CAD build for the part. Positions are in the model's coordinates, mm. A direction names the side the tool comes from. Coordinates: 2 decimals unless noted, no trailing zeros. Write each loop counter-clockwise with the first axis right and the second up, starting at its lowest first coordinate (ties: lowest second). Pieces come first, ordered by that corner, then holes. Notation, with made-up numbers: (-14, 72.25) - (35, 72.25) arc R21 ccw to (35, 78.25) - close; hole circle Ø6 at (65.5, -5). An arc over 180 degrees is marked (long way). Answer in a Markdown table with one row per item. Add a question column.
Q1. Band-saw the part on C-C (x = 26). List the corners of the cut face in (y, z).
Q2. Band-saw the part on D-D (z = -22). List the corners of the cut face in (x, y).
Q3. 3-axis set-ups, long thin cutter, end or side, ignore diameter. For faces 1 (the flat face through (-1, -20, 1)), 2 (the flat face through (-1, 0, -39.5)): which of +Z, -Z, +X, -X, +Y, -Y reach the whole face in a straight line?
Q4. Two-plate mould, pull along Z, no slides. Class faces 3 (the flat face through (1, 3, -5)), 4 (the flat face through (1, 0, 75)), 5 (the cylindrical face through (-0.651, -10.14, -40.043)), 6 (the flat face through (75, -5, 16)): +Z half, -Z half, draft (parallel to the pull), parting line (faces both ways), or undercut.
Q5. Drill centre lines: line 1 along Z through (x, y) = (0, -4); line 2 along Z through (x, y) = (-27, 5); line 3 along Y through (x, z) = (-63, -50). Where is each one in solid material? Low to high. Write a range as from..to.
Q6. Band-saw the part on B-B (z = -45). List the corners of the cut face in (x, y), and give its area (3 significant figures).
Q7. Pin check, flat tips, straight feed: pin 1 (3 mm diameter, centred on x = 9, z = 7, fed in from +Y); pin 2 (1.7 mm diameter, centred on x = 28, y = 3, fed in from -Z). Stop position of each tip, or through.
Q8. Band-saw the part on A-A (x = 0). List the corners of the cut face in (y, z).
```python
from build123d import *

# Parameters (mm, degrees)
F0_W     = 150
F0_H     = 150
F1_DEPTH = 20
F2_W     = 150
F2_H     = 80
F3_DEPTH = 20
F5_DEPTH = 150.001
F6_R     = 5
F7_DEPTH = 40.001


# Not quite as in the source:
# - a feature names something its author has since deleted; it is built from what else it names


with BuildPart() as f1:
    # F0 (on Front) → F1 (new body)
    with BuildSketch(Plane.XZ):
        Rectangle(F0_W, F0_H)
    extrude(amount=F1_DEPTH)

    # F2 (on face) → F3 (join)
    with BuildSketch(Plane(origin=(0, 0, 0), x_dir=(-1, 0, 0), z_dir=(0, 1, 0))):
        with Locations((0, 35)):
            Rectangle(F2_W, F2_H)
    extrude(amount=F3_DEPTH)

    # F4 (on face) → F5 (cut, through all)
    with BuildSketch(Plane.YZ.offset(75)):
        Polygon((20, -5), (20, 75), (5.5873245001, -5), align=None)
    extrude(amount=-F5_DEPTH, mode=Mode.SUBTRACT)

    # F6 (on face) → F7 (cut, through all)
    with BuildSketch(Plane.XZ.offset(20)):
        with Locations((0, -45)):
            Circle(F6_R)
    extrude(amount=-F7_DEPTH, mode=Mode.SUBTRACT)


solid = f1.part
```
Checked values:
| question | item | result |
|---|---|---|
| 1 | outline | (-20, -75) - (0, -75) - (0, -5) - (5.59, -5) - (20, 75) - (-20, 75) - close |
| 2 | outline | (-75, -20) - (75, -20) - (75, 0) - (-75, 0) - close |
| 3 | face 1 | +Z, -Z, +X, -X, -Y |
| 3 | face 2 | -Z, +X, -X, +Y |
| 4 | face 3 | -Z half |
| 4 | face 4 | +Z half |
| 4 | face 5 | undercut |
| 4 | face 6 | draft |
| 5 | line 1 | z = -75..-50, -40..75 |
| 5 | line 2 | z = -5..75 |
| 5 | line 3 | y = -20..0 |
| 6 | outline | (-75, -20) - (-5, -20) - (-5, 0) - (-75, 0) - close; (5, -20) - (75, -20) - (75, 0) - (5, 0) - close |
| 6 | area | 2,800 mm² |
| 7 | pin 1 | stops at y = 8.02 |
| 7 | pin 2 | stops at z = -5 |
| 8 | outline | (-20, -75) - (0, -75) - (0, -50) - (-20, -50) - close; (-20, -40) - (0, -40) - (0, -5) - (5.59, -5) - (20, 75) - (-20, 75) - close |
